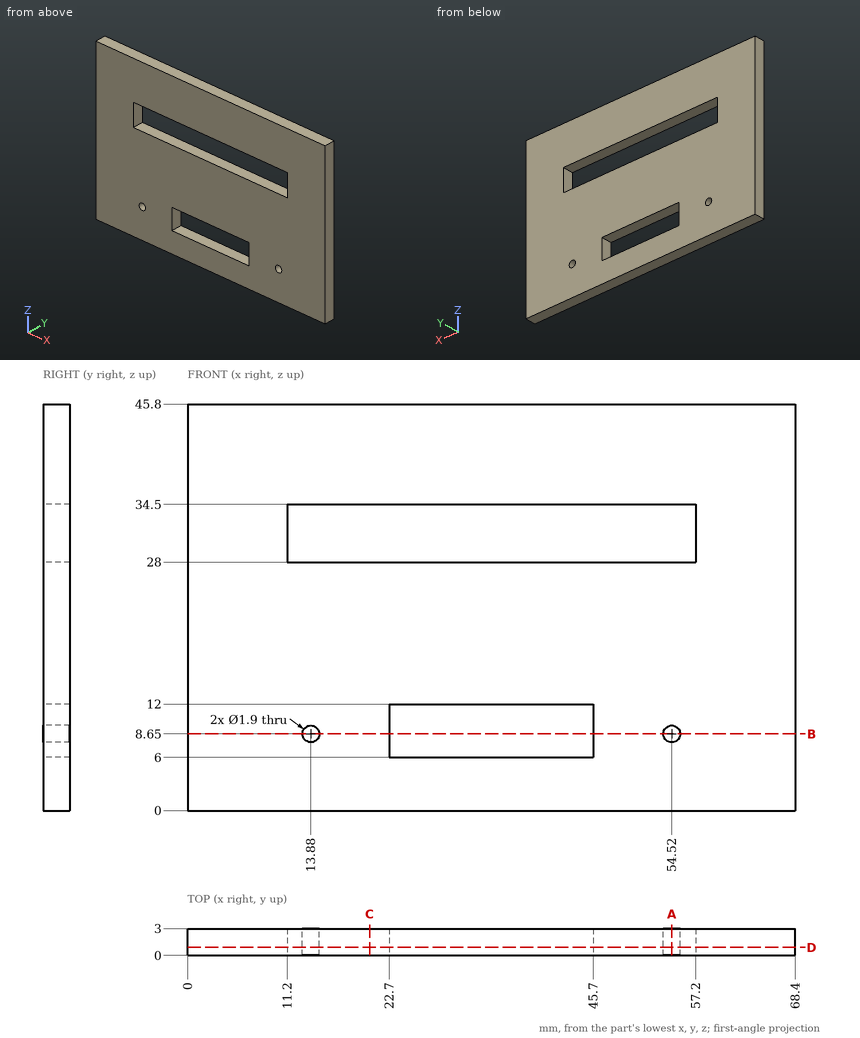
Design review of the part shown in the three views and the two pictorial views. Dimensions are in mm from the part's minimum x, y and z. Round coordinates to 2 decimals unless told otherwise and drop trailing zeros. Loops run counter-clockwise (first coordinate to the right, second up) from the corner with the lowest first, then second, coordinate; pieces in that order, holes last. Notation, with made-up numbers: (79, 18) - (112, 18) arc R14 ccw to (112, 25) - close; hole circle Ø9 at (1.25, 24). An arc over 180 degrees is marked (long way). Answer as CSV lines item,"result".
(1) Wall thickness on line 1 (X direction, y = 1.4, z = 8.65); line 2 (Z direction, x = 41, y = 2.2); line 3 (Z direction, x = 54.52, y = 0.9): over which ranges is each line inside the solid? List them lowest first.
Checked values:
line 1,"x = 0 to 12.93, 14.83 to 22.7, 45.7 to 53.57, 55.47 to 68.4"
line 2,"z = 0 to 6, 12 to 28, 34.5 to 45.8"
line 3,"z = 0 to 7.7, 9.6 to 28, 34.5 to 45.8"
(2) Consider section B-B on z = 8.65. Give the boundary of the cut face in (x, y).
Checked values:
outline,"(0, 0) - (12.93, 0) - (12.93, 3) - (0, 3) - close; (14.83, 0) - (22.7, 0) - (22.7, 3) - (14.83, 3) - close; (45.7, 0) - (53.57, 0) - (53.57, 3) - (45.7, 3) - close; (55.47, 0) - (68.4, 0) - (68.4, 3) - (55.47, 3) - close"
(3) Consider section D-D on y = 0.9. Give the boundary of the cut face in (x, z), then the cut area to 3 significant figures.
Checked values:
outline,"(0, 0) - (68.4, 0) - (68.4, 45.8) - (0, 45.8) - close; hole (11.2, 28) - (57.2, 28) - (57.2, 34.5) - (11.2, 34.5) - close; hole circle Ø1.9 at (13.88, 8.65); hole (22.7, 6) - (45.7, 6) - (45.7, 12) - (22.7, 12) - close; hole circle Ø1.9 at (54.52, 8.65)"
area,"2,690 mm2"
(4) Insertion check: P1, Ø1.5, axis at y = 1, z = 8.5, coming from the -X side. The pin has a flat end and moves straight along its axis. Give the tip position at first contact, or say it passes through.
Checked values:
P1,"stops at x = 0"
(5) Consider section A-A on x = 54.52. Give the boundary of the cut face in (y, z).
Checked values:
outline,"(0, 0) - (3, 0) - (3, 7.7) - (0, 7.7) - close; (0, 9.6) - (3, 9.6) - (3, 28) - (0, 28) - close; (0, 34.5) - (3, 34.5) - (3, 45.8) - (0, 45.8) - close"
(6) Consider section C-C on x = 20.5. Give the boundary of the cut face in (y, z), then the cut area to 3 significant figures.
Checked values:
outline,"(0, 0) - (3, 0) - (3, 28) - (0, 28) - close; (0, 34.5) - (3, 34.5) - (3, 45.8) - (0, 45.8) - close"
area,"118 mm2"
